The listing builds one solid part. Answer for the finished solid, in the listing's coordinates (mm). A direction names the side the tool comes from. Give positions to 0.01 mm unless a question says otherwise; leave off trailing zeros. Order: outer loops, then holes, each group sorted by start corner. A loop starts at its lowest first (then second) coordinate and runs counter-clockwise, first axis right, second up. Notation, with made-up numbers: (21.25, 41.5) - (34.25, 41.5) arc R10 ccw to (34.25, 57.5) - close; hole circle Ø4 at (15, 13.25). An arc over 180 degrees is marked (long way). Answer as a JSON object with one key per item and string values. Group by question number.
Q1. A cutting plane is placed at A-A, the plane z = -4. Count the separate pieces of the cut face and the enclosed holes in it, and give its area (3 significant figures).
Q2. For faces 1 (the face through (363, 65, 2)), 2 (the face through (384.8, 79, -8)), determine the directions among +Z, -Z, +X, -X, +Y, -Y from which every point of the face is accessible in a straight line to the end or side of a thin tool.
Q3. A cutting plane is placed at D-D, the plane x = 289. Give the vertices of the cut face in (y, z).
Q4. Given pin 1 (1 mm diameter, centred on x = 247, y = 88, fed in from +Z); pin 2 (9.5 mm diameter, centred on y = 76, z = 5, fed in from +X); pin 3 (3.5 mm diameter, centred on y = 76, z = 7, fed in from -X); pin 4 (1.8 mm diameter, centred on x = 259.8, y = 7, fed in from +Z), each flat-ended and moving along its own axis, determine where each tip first touches the part or whether it passes through.
Q5. Consider line 1 (Y direction, x = 259.8, z = -10); line 2 (Y direction, x = 364, z = -6); line 3 (Y direction, x = 231.8, z = -3.5). Determine where each line is inside the solid, lowest interval first.
Q6. The mould has two halves that part along X. Classify faces 3 (the face through (278.2, 150.8, 4.4)), 4 (the face through (363, 79, 15)), 5 (the face through (293, 80, 2)): released by +X, released by -X, zero draft, split by the parting line, or undercut.
Q7. A cutting plane is placed at B-B, the plane z = 13. Give the vertices of the cut face in (x, y).
Q8. A cutting plane is placed at C-C, the plane y = 26. Give the vertices of the cut face in (x, z).
from build123d import *

# Parameters (mm, degrees)
CYLINDER009_R     = 2
CYLINDER009_DEPTH = 10
FILLET_R          = 1
CYLINDER008_R     = 2
CYLINDER008_DEPTH = 10
FILLET001_R       = 1
BOX002_W          = 16
BOX002_H          = 12
BOX002_DEPTH      = 26
BOX003_W          = 13
BOX003_H          = 28
BOX003_DEPTH      = 26
CYLINDER_R        = 1.5
CYLINDER_DEPTH    = 16
CYLINDER001_R     = 1.5
CYLINDER001_DEPTH = 16
CYLINDER002_R     = 1.5
CYLINDER002_DEPTH = 16
CYLINDER003_R     = 1.5
CYLINDER003_DEPTH = 16
CYLINDER004_R     = 1.5
CYLINDER004_DEPTH = 16
CYLINDER005_R     = 1.5
CYLINDER005_DEPTH = 16
CYLINDER006_R     = 1.5
CYLINDER006_DEPTH = 16
CYLINDER007_R     = 1.5
CYLINDER007_DEPTH = 16
BOX001_W          = 132
BOX001_H          = 132
BOX001_DEPTH      = 11
BOX_W             = 160
BOX_H             = 160
BOX_DEPTH         = 16


with BuildPart() as fillet_body:
    # Cylinder009 → Cylinder009 (new body)
    with BuildSketch(Plane(origin=(55, 152, 16), x_dir=(1, 0, 0), z_dir=(0, 0, 1))):
        Circle(CYLINDER009_R)
    extrude(amount=CYLINDER009_DEPTH)

    # Fillet
    fillet_edges = [fillet_body.edges().sort_by_distance(p)[0] for p in [
        (53, 152, 26),
    ]]
    fillet(fillet_edges, radius=FILLET_R)


with BuildPart() as fillet001:
    # Cylinder008 → Cylinder008 (new body)
    with BuildSketch(Plane(origin=(105, 7, 16), x_dir=(1, 0, 0), z_dir=(0, 0, 1))):
        Circle(CYLINDER008_R)
    extrude(amount=CYLINDER008_DEPTH)

    # Fillet001
    fillet001_edges = [fillet001.edges().sort_by_distance(p)[0] for p in [
        (103, 7, 26),
    ]]
    fillet(fillet001_edges, radius=FILLET001_R)


with BuildPart() as cube002:
    # Box002 → Box002 (new body)
    with BuildSketch(Plane(origin=(60, 68, 5), x_dir=(1, 0, 0), z_dir=(0, 0, 1))):
        with Locations((8, 6)):
            Rectangle(BOX002_W, BOX002_H)
    extrude(amount=BOX002_DEPTH)


with BuildPart() as cube003:
    # Box003 → Box003 (new body)
    with BuildSketch(Plane(origin=(132, 65, 5), x_dir=(1, 0, 0), z_dir=(0, 0, 1))):
        with Locations((6.5, 14)):
            Rectangle(BOX003_W, BOX003_H)
    extrude(amount=BOX003_DEPTH)


with BuildPart() as cylinder:
    # Cylinder → Cylinder (new body)
    with BuildSketch(Plane(origin=(35, 7, 0), x_dir=(1, 0, 0), z_dir=(0, 0, 1))):
        Circle(CYLINDER_R)
    extrude(amount=CYLINDER_DEPTH)


with BuildPart() as cylinder001:
    # Cylinder001 → Cylinder001 (new body)
    with BuildSketch(Plane(origin=(124.5, 7, 0), x_dir=(1, 0, 0), z_dir=(0, 0, 1))):
        Circle(CYLINDER001_R)
    extrude(amount=CYLINDER001_DEPTH)


with BuildPart() as cylinder002:
    # Cylinder002 → Cylinder002 (new body)
    with BuildSketch(Plane(origin=(35, 152, 0), x_dir=(1, 0, 0), z_dir=(0, 0, 1))):
        Circle(CYLINDER002_R)
    extrude(amount=CYLINDER002_DEPTH)


with BuildPart() as cylinder003:
    # Cylinder003 → Cylinder003 (new body)
    with BuildSketch(Plane(origin=(124.5, 152, 0), x_dir=(1, 0, 0), z_dir=(0, 0, 1))):
        Circle(CYLINDER003_R)
    extrude(amount=CYLINDER003_DEPTH)


with BuildPart() as cylinder004:
    # Cylinder004 → Cylinder004 (new body)
    with BuildSketch(Plane(origin=(7, 30, 0), x_dir=(1, 0, 0), z_dir=(0, 0, 1))):
        Circle(CYLINDER004_R)
    extrude(amount=CYLINDER004_DEPTH)


with BuildPart() as cylinder005:
    # Cylinder005 → Cylinder005 (new body)
    with BuildSketch(Plane(origin=(7, 130, 0), x_dir=(1, 0, 0), z_dir=(0, 0, 1))):
        Circle(CYLINDER005_R)
    extrude(amount=CYLINDER005_DEPTH)


with BuildPart() as cylinder006:
    # Cylinder006 → Cylinder006 (new body)
    with BuildSketch(Plane(origin=(152, 30, 0), x_dir=(1, 0, 0), z_dir=(0, 0, 1))):
        Circle(CYLINDER006_R)
    extrude(amount=CYLINDER006_DEPTH)


with BuildPart() as anchor_holes:
    # Cylinder007 → Cylinder007 (new body)
    with BuildSketch(Plane(origin=(152, 130, 0), x_dir=(1, 0, 0), z_dir=(0, 0, 1))):
        Circle(CYLINDER007_R)
    extrude(amount=CYLINDER007_DEPTH)

    # Fusion: union Cylinder, Cylinder001, Cylinder002, Cylinder003, Cylinder004, Cylinder005, Cylinder006
    add(cylinder.part)
    add(cylinder001.part)
    add(cylinder002.part)
    add(cylinder003.part)
    add(cylinder004.part)
    add(cylinder005.part)
    add(cylinder006.part)


with BuildPart() as cube001:
    # Box001 → Box001 (new body)
    with BuildSketch(Plane(origin=(14, 14, 5), x_dir=(1, 0, 0), z_dir=(0, 0, 1))):
        with Locations((66, 66)):
            Rectangle(BOX001_W, BOX001_H)
    extrude(amount=BOX001_DEPTH)


with BuildPart() as led_array:
    # Box → Box (new body)
    with BuildSketch(Plane.XY):
        with Locations((80, 80)):
            Rectangle(BOX_W, BOX_H)
    extrude(amount=BOX_DEPTH)

    # Cut: cut Cube001
    add(cube001.part, mode=Mode.SUBTRACT)

    # Cut001: cut Anchor Holes
    add(anchor_holes.part, mode=Mode.SUBTRACT)

    # Fusion001: union Cube002, Cube003
    add(cube002.part)
    add(cube003.part)

    # Fusion002: union Fillet body, Fillet001
    add(fillet_body.part)
    add(fillet001.part)


with BuildPart() as led_array_1:
    # Fusion002 placement: moved
    add(led_array.part.moved(Location((224.8, 0, -16))))


solid = led_array_1.part
Reply:
{
 "1": {"separate pieces": "3", "enclosed holes": "9", "area": "8,680 mm^2"},
 "2": {"face 1": "+Z", "face 2": "+Z, -Z, +X, +Y, -Y"},
 "3": {"outline": "(0, -16) - (160, -16) - (160, 0) - (146, 0) - (146, -11) - (80, -11) - (80, 15) - (68, 15) - (68, -11) - (14, -11) - (14, 0) - (0, 0) - close"},
 "4": {"pin 1": "stops at z = -11", "pin 2": "stops at x = 369.8", "pin 3": "stops at x = 284.8", "pin 4": "passes through"},
 "5": {"line 1": "y = 0 to 5.5, 8.5 to 14, 146 to 150.5, 153.5 to 160", "line 2": "y = 0 to 14, 65 to 93, 146 to 160", "line 3": "y = 0 to 28.5, 31.5 to 128.5, 131.5 to 160"},
 "6": {"face 3": "split by the parting line", "face 4": "zero draft", "face 5": "undercut"},
 "7": {"outline": "(284.8, 68) - (300.8, 68) - (300.8, 80) - (284.8, 80) - close; (356.8, 65) - (369.8, 65) - (369.8, 93) - (356.8, 93) - close"},
 "8": {"outline": "(224.8, -16) - (384.8, -16) - (384.8, 0) - (370.8, 0) - (370.8, -11) - (238.8, -11) - (238.8, 0) - (224.8, 0) - close"}
}
